Work out the finished part from the listing and answer in its coordinate system (mm). Round coordinates to 2 decimals unless told otherwise and drop trailing zeros. Order: outer loops, then holes, each group sorted by start corner. A loop starts at its lowest first (then second) coordinate and runs counter-clockwise, first axis right, second up. Notation, with made-up numbers: (26, 73) - (58, 73) arc R31 ccw to (58, 111) - close; hole circle Ø9 at (29, 31). An arc over 180 degrees is marked (long way). Use CSV: the item, a comma, the result in double quotes.
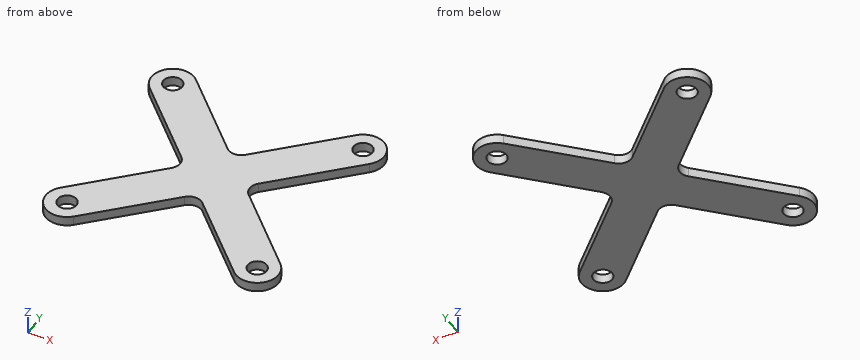
from build123d import *

# Parameters (mm, degrees)
F0_R     = 1.5
F1_DEPTH = 1.5


with BuildPart() as f1:
    # F0 (on Top) → F1 (new body)
    with BuildSketch(Plane.XY):
        with BuildLine():
            ThreePointArc((-12.863515, 17.636485), (-17.636485, 17.636485), (-17.636485, 12.863515))
            Line((-17.636485, 12.863515), (-6.187184, 1.414214))
            ThreePointArc((-6.187184, 1.414214), (-5.601398, 0), (-6.187184, -1.414214))
            Line((-6.187184, -1.414214), (-17.636485, -12.863515))
            ThreePointArc((-17.636485, -12.863515), (-17.636485, -17.636485), (-12.863515, -17.636485))
            Line((-12.863515, -17.636485), (-1.414214, -6.187184))
            ThreePointArc((-1.414214, -6.187184), (0, -5.601398), (1.414214, -6.187184))
            Line((1.414214, -6.187184), (12.863515, -17.636485))
            ThreePointArc((12.863515, -17.636485), (17.636485, -17.636485), (17.636485, -12.863515))
            Line((17.636485, -12.863515), (6.187184, -1.414214))
            ThreePointArc((6.187184, -1.414214), (5.601398, 0), (6.187184, 1.414214))
            Line((6.187184, 1.414214), (17.636485, 12.863515))
            ThreePointArc((17.636485, 12.863515), (17.636485, 17.636485), (12.863515, 17.636485))
            Line((12.863515, 17.636485), (1.414214, 6.187184))
            ThreePointArc((1.414214, 6.187184), (0, 5.601398), (-1.414214, 6.187184))
            Line((-1.414214, 6.187184), (-12.863515, 17.636485))
        make_face()
        with Locations((-15.25, -15.25)):
            Circle(F0_R, mode=Mode.SUBTRACT)
        with Locations((15.25, -15.25)):
            Circle(F0_R, mode=Mode.SUBTRACT)
        with Locations((-15.25, 15.25)):
            Circle(F0_R, mode=Mode.SUBTRACT)
        with Locations((15.25, 15.25)):
            Circle(F0_R, mode=Mode.SUBTRACT)
    extrude(amount=F1_DEPTH)


solid = f1.part
(1) Find section D-D (x = 15.25). Determine the outline of the cut face in (y, z) (3 decimals).
Findings below:
outline,"(-18.625, 0) - (-16.75, 0) - (-16.75, 1.5) - (-18.625, 1.5) - close; (-13.75, 0) - (-10.477, 0) - (-10.477, 1.5) - (-13.75, 1.5) - close; (10.477, 0) - (13.75, 0) - (13.75, 1.5) - (10.477, 1.5) - close; (16.75, 0) - (18.625, 0) - (18.625, 1.5) - (16.75, 1.5) - close"
(2) Find the intervals of material crossed by L1, parallel to Y at x = -15, z = 0.85; L2, parallel to Y at x = 15.25, z = 0.8 (3 decimals); L3, parallel to X at y = 13, z = 0.95, in increasing order. Write a range as from..to.
Findings below:
L1,"y = -18.62..-16.73, -13.77..-10.23, 10.23..13.77, 16.73..18.62"
L2,"y = -18.625..-16.75, -13.75..-10.477, 10.477..13.75, 16.75..18.625"
L3,"x = -17.77..-8.23, 8.23..17.77"
(3) Find section A-A (z = 1.2). Determine the outline of the cut face in (x, y) (3 decimals).
Findings below:
outline,"(-17.636, -12.864) arc R3.375 ccw to (-12.864, -17.636) - (-1.414, -6.187) arc R2 cw to (1.414, -6.187) - (12.864, -17.636) arc R3.375 ccw to (17.636, -12.864) - (6.187, -1.414) arc R2 cw to (6.187, 1.414) - (17.636, 12.864) arc R3.375 ccw to (12.864, 17.636) - (1.414, 6.187) arc R2 cw to (-1.414, 6.187) - (-12.864, 17.636) arc R3.375 ccw to (-17.636, 12.864) - (-6.187, 1.414) arc R2 cw to (-6.187, -1.414) - close; hole circle Ø3 at (-15.25, -15.25); hole circle Ø3 at (-15.25, 15.25); hole circle Ø3 at (15.25, -15.25); hole circle Ø3 at (15.25, 15.25)"
(4) Find section B-B (y = 11.5). Determine the outline of the cut face in (x, z), and give its area (3 significant figures).
Findings below:
outline,"(-16.27, 0) - (-6.73, 0) - (-6.73, 1.5) - (-16.27, 1.5) - close; (6.73, 0) - (16.27, 0) - (16.27, 1.5) - (6.73, 1.5) - close"
area,"28.6 mm²"
(5) Find section C-C (x = 9). Determine the outline of the cut face in (y, z).
Findings below:
outline,"(-13.77, 0) - (-4.23, 0) - (-4.23, 1.5) - (-13.77, 1.5) - close; (4.23, 0) - (13.77, 0) - (13.77, 1.5) - (4.23, 1.5) - close"
(6) This flat-tipped pin is pushed along its axis until it touches: pin 1 (3.5 mm diameter, centred on x = 15.25, y = -15.25, fed in from -Z). Where does it stop, or does it pass through?
Findings below:
pin 1,"stops at z = 0"
